```python
from build123d import *

# Parameters (mm, degrees)
BOSS_EXTRUDE1_DEPTH = 16
SKETCH2_R           = 1.275
CUT_EXTRUDE1_DEPTH  = 18.471332994


with BuildPart() as part:
    # Sketch1 → Boss-Extrude1 (new body)
    with BuildSketch(Plane(origin=(0, 0, 0), x_dir=(1, 0, 0), z_dir=(0, 1, 0))):
        with BuildLine():
            Line((-0.25, 4.993746089), (-0.476626074, 3.971501931))
            ThreePointArc((-0.476626074, 3.971501931), (-0.890083736, 3.899711649), (-1.293744854, 3.784999901))
            Line((-1.293744854, 3.784999901), (-1.941463008, 4.607680695))
            ThreePointArc((-1.941463008, 4.607680695), (-2.169418696, 4.50484434), (-2.391947442, 4.390738825))
            Line((-2.391947442, 4.390738825), (-2.152595362, 3.371399295))
            ThreePointArc((-2.152595362, 3.371399295), (-2.493959207, 3.12732593), (-2.807873746, 2.848832222))
            Line((-2.807873746, 2.848832222), (-3.748395457, 3.30900763))
            ThreePointArc((-3.748395457, 3.30900763), (-3.909157412, 3.117449009), (-4.060140358, 2.918091889))
            Line((-4.060140358, 2.918091889), (-3.402216738, 2.103549682))
            ThreePointArc((-3.402216738, 2.103549682), (-3.603875472, 1.735534956), (-3.765868806, 1.348418382))
            Line((-3.765868806, 1.348418382), (-4.812912215, 1.354945022))
            ThreePointArc((-4.812912215, 1.354945022), (-4.874639561, 1.11260467), (-4.924172682, 0.867481066))
            Line((-4.924172682, 0.867481066), (-3.977987365, 0.419066256))
            ThreePointArc((-3.977987365, 0.419066256), (-4, 0), (-3.977987365, -0.419066256))
            Line((-3.977987365, -0.419066256), (-4.924172682, -0.867481066))
            ThreePointArc((-4.924172682, -0.867481066), (-4.874639561, -1.11260467), (-4.812912215, -1.354945022))
            Line((-4.812912215, -1.354945022), (-3.765868806, -1.348418382))
            ThreePointArc((-3.765868806, -1.348418382), (-3.603875472, -1.735534956), (-3.402216738, -2.103549682))
            Line((-3.402216738, -2.103549682), (-4.060140358, -2.918091889))
            ThreePointArc((-4.060140358, -2.918091889), (-3.909157412, -3.117449009), (-3.748395457, -3.30900763))
            Line((-3.748395457, -3.30900763), (-2.807873746, -2.848832222))
            ThreePointArc((-2.807873746, -2.848832222), (-2.493959207, -3.12732593), (-2.152595362, -3.371399295))
            Line((-2.152595362, -3.371399295), (-2.391947442, -4.390738825))
            ThreePointArc((-2.391947442, -4.390738825), (-2.169418696, -4.50484434), (-1.941463008, -4.607680695))
            Line((-1.941463008, -4.607680695), (-1.293744854, -3.784999901))
            ThreePointArc((-1.293744854, -3.784999901), (-0.890083736, -3.899711649), (-0.476626074, -3.971501931))
            Line((-0.476626074, -3.971501931), (-0.25, -4.993746089))
            ThreePointArc((-0.25, -4.993746089), (0, -5), (0.25, -4.993746089))
            Line((0.25, -4.993746089), (0.476626074, -3.971501931))
            ThreePointArc((0.476626074, -3.971501931), (0.890083736, -3.899711649), (1.293744854, -3.784999901))
            Line((1.293744854, -3.784999901), (1.941463008, -4.607680695))
            ThreePointArc((1.941463008, -4.607680695), (2.169418696, -4.50484434), (2.391947442, -4.390738825))
            Line((2.391947442, -4.390738825), (2.152595362, -3.371399295))
            ThreePointArc((2.152595362, -3.371399295), (2.493959207, -3.12732593), (2.807873746, -2.848832222))
            Line((2.807873746, -2.848832222), (3.748395457, -3.30900763))
            ThreePointArc((3.748395457, -3.30900763), (3.909157412, -3.117449009), (4.060140358, -2.918091889))
            Line((4.060140358, -2.918091889), (3.402216738, -2.103549682))
            ThreePointArc((3.402216738, -2.103549682), (3.603875472, -1.735534956), (3.765868806, -1.348418382))
            Line((3.765868806, -1.348418382), (4.812912215, -1.354945022))
            ThreePointArc((4.812912215, -1.354945022), (4.874639561, -1.11260467), (4.924172682, -0.867481066))
            Line((4.924172682, -0.867481066), (3.977987365, -0.419066256))
            ThreePointArc((3.977987365, -0.419066256), (4, 0), (3.977987365, 0.419066256))
            Line((3.977987365, 0.419066256), (4.924172682, 0.867481066))
            ThreePointArc((4.924172682, 0.867481066), (4.874639561, 1.11260467), (4.812912215, 1.354945022))
            Line((4.812912215, 1.354945022), (3.765868806, 1.348418382))
            ThreePointArc((3.765868806, 1.348418382), (3.603875472, 1.735534956), (3.402216738, 2.103549682))
            Line((3.402216738, 2.103549682), (4.060140358, 2.918091889))
            ThreePointArc((4.060140358, 2.918091889), (3.909157412, 3.117449009), (3.748395457, 3.30900763))
            Line((3.748395457, 3.30900763), (2.807873746, 2.848832222))
            ThreePointArc((2.807873746, 2.848832222), (2.493959207, 3.12732593), (2.152595362, 3.371399295))
            Line((2.152595362, 3.371399295), (2.391947442, 4.390738825))
            ThreePointArc((2.391947442, 4.390738825), (2.169418696, 4.50484434), (1.941463008, 4.607680695))
            Line((1.941463008, 4.607680695), (1.293744854, 3.784999901))
            ThreePointArc((1.293744854, 3.784999901), (0.890083736, 3.899711649), (0.476626074, 3.971501931))
            Line((0.476626074, 3.971501931), (0.25, 4.993746089))
            ThreePointArc((0.25, 4.993746089), (0, 5), (-0.25, 4.993746089))
        make_face()
    extrude(amount=BOSS_EXTRUDE1_DEPTH)

    # Sketch2 → Cut-Extrude1 (cut, through all)
    with BuildSketch(Plane.XZ):
        with Locations(Location((0, 0, 0), (0, 0, 270))):
            Circle(SKETCH2_R)
    extrude(amount=-CUT_EXTRUDE1_DEPTH, mode=Mode.SUBTRACT)


solid = part.part
```
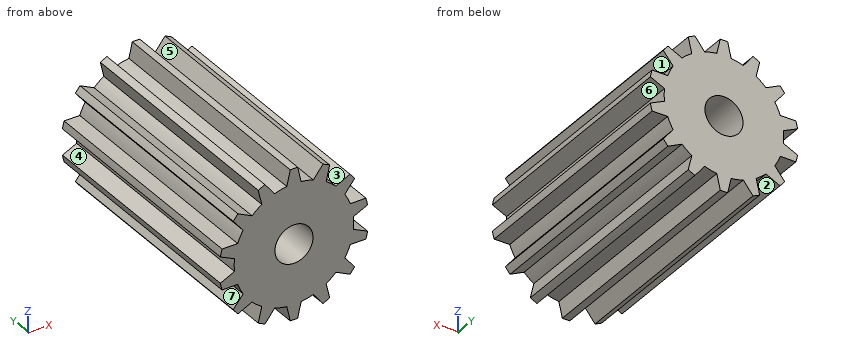
For this review, take the finished solid that the model builds, in its own axes (mm). Face numbers are marked on the shaded views. A direction names the side the tool comes from. Round coordinates to 2 decimals unless told otherwise and drop trailing zeros. Order: outer loops, then holes, each group sorted by start corner. A loop starts at its lowest first (then second) coordinate and runs counter-clockwise, first axis right, second up. Notation, with made-up numbers: (57, 33) -> (100, 33) arc R15 ccw to (100, 52) -> close; hole circle Ø11 at (78, 51). An arc over 180 degrees is marked (long way). Use a Markdown table: item, result.
Item 1: For pin 1 (1 mm diameter, centred on y = 4.5, z = -2.5, fed in from -X); pin 2 (4 mm diameter, centred on y = 2.5, z = -2, fed in from +X); pin 3 (1.5 mm diameter, centred on x = 0, z = 0, fed in from +Y), all flat-tipped, find the tip position at first contact; note any pin that passes through.
Resolved:
| item | result |
|---|---|
| pin 1 | stops at x = -4.06 |
| pin 2 | stops at x = 4.92 |
| pin 3 | passes through |
Item 2: For line 1 along X through (y, z) = (7.75, 0) (3 decimals); line 2 along X through (y, z) = (2.5, -4.5); line 3 along Z through (x, y) = (1, 12.75), list the stretches that pass through material, from the lowest coordinate up. Write a range as [from, to].
Resolved:
| item | result |
|---|---|
| line 1 | x = [-4, -1.275], [1.275, 4] |
| line 2 | x = [-2.18, -1.86], [-0.36, 0.36], [1.86, 2.18] |
| line 3 | z = [-3.87, -0.79], [0.79, 3.87] |
Item 3: Take a section at D-D (x = 3). State the section outline as (y, z) points.
Resolved:
| item | result |
|---|---|
| outline | (0, -2.94) -> (16, -2.94) -> (16, 2.94) -> (0, 2.94) -> close |
Item 4: Machinability: for the marked faces 1, 2, 3 and 4, which of the approach directions +Z, -Z, +X, -X, +Y, -Y give a long, thin tool a straight path to every point of the face, cutting with its end or side? Answer none if there is none.
Resolved:
| item | result |
|---|---|
| face 1 | +X, +Y, -Y |
| face 2 | -Z, +Y, -Y |
| face 3 | +Z, +Y, -Y |
| face 4 | -X, +Y, -Y |
Item 5: Draft analysis for pull direction X (two halves, no side actions). For the marked faces 5, 6 and 7, state which applies: +X half, -X half, draft (parallel to the pull), parting line (faces both ways), or undercut.
Resolved:
| item | result |
|---|---|
| face 5 | undercut |
| face 6 | +X half |
| face 7 | -X half |
Item 6: Take a section at C-C (x = -1.75). State the section outline as (y, z) points, plus the area to 3 significant figures.
Resolved:
| item | result |
|---|---|
| outline | (0, -4.36) -> (16, -4.36) -> (16, 4.36) -> (0, 4.36) -> close |
| area | 140 mm² |
Item 7: Take a section at B-B (x = 0). State the section outline as (y, z) points (3 decimals).
Resolved:
| item | result |
|---|---|
| outline | (0, -5) -> (16, -5) -> (16, -1.275) -> (0, -1.275) -> close; (0, 1.275) -> (16, 1.275) -> (16, 5) -> (0, 5) -> close |
Item 8: Take a section at A-A (z = 0). State the section outline as (x, y) points (3 decimals), plus the area to 3 significant figures.
Resolved:
| item | result |
|---|---|
| outline | (-4, 0) -> (-1.275, 0) -> (-1.275, 16) -> (-4, 16) -> close; (1.275, 0) -> (4, 0) -> (4, 16) -> (1.275, 16) -> close |
| area | 87.2 mm² |
